Source: CAD feature listing. Evaluate the final solid. Frame: model axes, mm. A direction names the side the tool comes from. Round coordinates to 2 decimals unless told otherwise and drop trailing zeros. Order: outer loops, then holes, each group sorted by start corner. A loop starts at its lowest first (then second) coordinate and runs counter-clockwise, first axis right, second up. Notation, with made-up numbers: M -31,6.5 L -21,6.5 A23 cw -21,26.5 Z; hole C 42.5,-35 d5. An arc over 180 degrees is marked long. Use one line per item in the form item = value. Start each with the question number.
Q1. Contact query for flat-ended pins moving along their axis: pin 1 (5 mm diameter, centred on x = -14, y = 2.5, fed in from +Z); pin 2 (2 mm diameter, centred on y = -3.5, z = 3.5, fed in from -X); pin 3 (4 mm diameter, centred on y = -2, z = -1, fed in from +X). Output: stop coordinate, or through.
Q2. Section B-B (y = 0). Return the cut outline in (x, z), plus the area to 3 significant figures.
Q3. Section A-A (z = 0). Return the cut outline in (x, y), plus the area to 3 significant figures.
Q4. Section C-C (x = 5). Return the cut outline in (y, z), plus the area to 3 significant figures.
Q5. Pull-direction query (Y, two-part tool) for faces 1 (the cylindrical face through (-16.18, -3.905, 0.867)), 2 (the cylindrical face through (4.2, -3.6, 4.5)), 3 (the flat face through (-16.5, -1, 2)); classes: pulls with the +Y half, pulls with the -Y half, needs draft (parallel to the pull), parting line crosses it, or undercut.
Q6. Material intervals for probe 1 along X at (y, z) = (-2, -2.25); probe 2 along X at (y, z) = (5, -0.75); probe 3 along Y at (x, z) = (-5, 5.45), sorted ascending.
Q7. Section D-D (y = 3). Return the cut outline in (x, z).
Q8. Reachability of faces 4 (the cylindrical face through (11.11, 0.03, 0.75)), 5 (the cylindrical face through (-13, -2, 0)), 6 (the flat face through (-5, 3, 3)), 7 (the cylindrical face through (-17, -2, 0)), 8 (the flat face through (0, 0, -6)) from +Z, -Z, +X, -X, +Y, -Y: full face, straight path, thin tool, end or side. Return the list, or none.
from build123d import *

# Parameters (mm, degrees)
SKETCH1_W           = 20
SKETCH1_H           = 12
BOSS_EXTRUDE1_DEPTH = 5.5
SKETCH2_R           = 1
CUT_EXTRUDE1_DEPTH  = 3


with BuildPart() as part:
    # Sketch1 → Boss-Extrude1 (new body, symmetric)
    with BuildSketch(Plane(origin=(0, 0, 0), x_dir=(1, 0, 0), z_dir=(0, 1, 0))):
        Rectangle(SKETCH1_W, SKETCH1_H)
    extrude(amount=BOSS_EXTRUDE1_DEPTH, both=True)

    # Sketch2 → Cut-Extrude1 (cut)
    with BuildSketch(Plane.XY.offset(6)):
        with Locations((5, -3)):
            Circle(SKETCH2_R)
        with Locations((-5, 3)):
            Circle(SKETCH2_R)
    extrude(amount=-CUT_EXTRUDE1_DEPTH, mode=Mode.SUBTRACT)

    # Sketch3 → Revolve1 (revolve)
    with BuildSketch(Plane(origin=(0, 0, 0), x_dir=(1, 0, 0), z_dir=(0, 1, 0))):
        Polygon((12, 0), (12, 0.75), (10.25, 0.75), (10.25, 1.566987298), (10, 2), (-15.85, 2), (-15.85, 4), (-16.5, 4), (-16.5, 2), (-17.5, 2), (-17.5, 0), align=None)
    revolve(axis=Axis((-17.5, 0, 0), (1, 0, 0)))


solid = part.part
Results list:
q1.pin_1 = 3.92
q1.pin_2 = -16.5
q1.pin_3 = 12
q2.outline = M -17.5,-2 L -16.5,-2 L -16.5,-4 L -15.85,-4 L -15.85,-2 L -10,-2 L -10,-6 L 10,-6 L 10,-2 L 10.25,-1.57 L 10.25,-0.75 L 12,-0.75 L 12,0.75 L 10.25,0.75 L 10.25,1.57 L 10,2 L 10,6 L -10,6 L -10,2 L -15.85,2 L -15.85,4 L -16.5,4 L -16.5,2 L -17.5,2 Z
q2.area = 276 mm2
q3.outline = M -17.5,-2 L -16.5,-2 L -16.5,-4 L -15.85,-4 L -15.85,-2 L -10,-2 L -10,-5.5 L 10,-5.5 L 10,-2 L 10.25,-1.57 L 10.25,-0.75 L 12,-0.75 L 12,0.75 L 10.25,0.75 L 10.25,1.57 L 10,2 L 10,5.5 L -10,5.5 L -10,2 L -15.85,2 L -15.85,4 L -16.5,4 L -16.5,2 L -17.5,2 Z
q3.area = 256 mm2
q4.outline = M -5.5,-6 L 5.5,-6 L 5.5,6 L -2,6 L -2,3 L -4,3 L -4,6 L -5.5,6 Z
q4.area = 126 mm2
q5.face_1 = parting line crosses it
q5.face_2 = undercut
q5.face_3 = needs draft
q6.probe_1 = -16.5 to -15.85, -10 to 10
q6.probe_2 = -10 to 10
q6.probe_3 = -5.5 to 2, 4 to 5.5
q7.outline = M -16.5,-2.65 L -15.85,-2.65 L -15.85,2.65 L -16.5,2.65 Z; M -10,-6 L 10,-6 L 10,6 L -4,6 L -4,3 L -6,3 L -6,6 L -10,6 Z
q8.face_4 = +X
q8.face_5 = none
q8.face_6 = +Z
q8.face_7 = -X
q8.face_8 = -Z, +X, -X, +Y, -Y
